Read the model definition and answer for the solid it produces. Units are mm, in the model's axes. Face numbers are marked on the shaded views. A direction names the side the tool comes from. Coordinates: 2 decimals unless noted, no trailing zeros. Loops run counter-clockwise (first coordinate to the right, second up) from the corner with the lowest first, then second, coordinate; pieces in that order, holes last. Notation, with made-up numbers: (8, 50.25) - (34, 50.25) arc R12 cw to (34, 69.25) - close; hole circle Ø5 at (18.5, 65.5). An arc over 180 degrees is marked (long way). Use one line per item in the form item = value.
from build123d import *

# Parameters (mm, degrees)
F0_R     = 12.5
F1_DEPTH = 45
F2_R     = 9.5
F3_DEPTH = 57
F4_R     = 6
F5_DEPTH = 15
F6_DEPTH = 40


with BuildPart() as f1:
    # F0 (on Right) → F1 (new body)
    with BuildSketch(Plane.YZ):
        Circle(F0_R)
    extrude(amount=F1_DEPTH)

    # F2 (on face) → F3 (join)
    with BuildSketch(Plane.YZ.offset(45)):
        Circle(F2_R)
    extrude(amount=F3_DEPTH)

    # F4 (on face) → F5 (join)
    with BuildSketch(Plane.YZ.offset(102)):
        Circle(F4_R)
    extrude(amount=F5_DEPTH)

    # F4 (on face) → F6 (cut, symmetric)
    with BuildSketch(Plane.YZ.offset(102)):
        with BuildLine():
            Line((0, 9.5), (0, 6.6651513899))
            Line((0, 6.6651513899), (2.5, 6.6651513899))
            Line((2.5, 6.6651513899), (2.5, 9.1651513899))
            ThreePointArc((2.5, 9.1651513899), (1.2611625184, 9.4159157336), (0, 9.5))
        make_face()
        with BuildLine():
            Line((-2.5, 9.1651513899), (-2.5, 6.6651513899))
            Line((-2.5, 6.6651513899), (0, 6.6651513899))
            Line((0, 6.6651513899), (0, 9.5))
            ThreePointArc((0, 9.5), (-1.2611625184, 9.4159157336), (-2.5, 9.1651513899))
        make_face()
    extrude(amount=F6_DEPTH, both=True, mode=Mode.SUBTRACT)


solid = f1.part
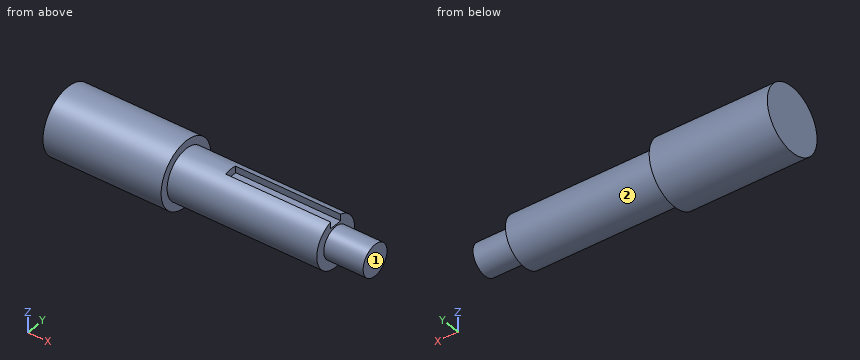
Item 1: The part is cut by section A-A on z = 0. Give the vertices of the cut face in (x, y), plus the area to 3 significant figures.
Results below:
outline = (0, -12.5) - (45, -12.5) - (45, -9.5) - (102, -9.5) - (102, -6) - (117, -6) - (117, 6) - (102, 6) - (102, 9.5) - (45, 9.5) - (45, 12.5) - (0, 12.5) - close
area = 2,390 mm²
Item 2: The part is cut by section D-D on y = -4.5. Give the vertices of the cut face in (x, z).
Results below:
outline = (0, -11.66) - (45, -11.66) - (45, -8.37) - (102, -8.37) - (102, -3.97) - (117, -3.97) - (117, 3.97) - (102, 3.97) - (102, 8.37) - (45, 8.37) - (45, 11.66) - (0, 11.66) - close
Item 3: Each of these flat-tipped pins is pushed along its axis until it touches: P1, Ø3, axis at x = 101.5, z = -3.5, coming from the +Y side; P2, Ø2, axis at x = 53.5, y = -7, coming from the -Z side; P3, Ø4, axis at x = 84.5, z = -8.5, coming from the +Y side. Where does it stop, or does it pass through?
Results below:
P1 = 9.29
P2 = -7.37
P3 = 6.93
Item 4: The part is cut by section C-C on x = 64. Give the vertices of the cut face in (y, z), plus the area to 3 significant figures.
Results below:
outline = (-2.5, 6.67) - (-2.5, 9.17) arc R9.5 ccw (long way) to (2.5, 9.17) - (2.5, 6.67) - close
area = 270 mm²
Item 5: Find the intervals of material crossed by L1, parallel to X at y = 1, z = 10.75; L2, parallel to Z at x = 18, y = 0.75; L3, parallel to Z at x = 71, y = 0, in increasing order.
Results below:
L1 = 0 to 45
L2 = -12.48 to 12.48
L3 = -9.5 to 6.67
Item 6: Which of the six approach directions +Z, -Z, +X, -X, +Y, -Y give full straight-line access (tool end or side, diameter ignored) to the marked faces 1 and 2?
Results below:
face_1 = +Z, -Z, +X, +Y, -Y
face_2 = +X
Item 7: The part is cut by section B-B on y = 0. Give the vertices of the cut face in (x, z), plus the area to 3 significant figures.
Results below:
outline = (0, -12.5) - (45, -12.5) - (45, -9.5) - (102, -9.5) - (102, -6) - (117, -6) - (117, 6) - (102, 6) - (102, 6.67) - (62, 6.67) - (62, 9.5) - (45, 9.5) - (45, 12.5) - (0, 12.5) - close
area = 2,270 mm²
